Part model, mm, in its own coordinate system. Round coordinates to 2 decimals unless told otherwise and drop trailing zeros. Loops run counter-clockwise (first coordinate to the right, second up) from the corner with the lowest first, then second, coordinate; pieces in that order, holes last. Notation, with made-up numbers: (25, 87) -> (53, 87) arc R19 ccw to (53, 109) -> close; hole circle Ø1 at (-39.75, -38). An arc over 180 degrees is marked (long way). Answer as a JSON object with one key per item and string values. Group by question number.
from build123d import *

# Parameters (mm, degrees)
SKETCH_1_W             = 112
SKETCH_1_H             = 110.77381068
SKETCH_1_R             = 5.25
SM_BASE_FLANGE_1_DEPTH = 6
CHAMFER_1_SIZE         = 15
CUT_EXTRUDE_1_DEPTH    = 10


# Sheet-metal steps are written as plain solids
with BuildPart() as part:
    # Sketch 1 → Базовая кромка1 (new body)
    with BuildSketch(Plane.XY):
        with Locations((0, 58.38690534)):
            Rectangle(SKETCH_1_W, SKETCH_1_H)
        with Locations((-28, 43)):
            Circle(SKETCH_1_R, mode=Mode.SUBTRACT)
        with Locations(Location((28, 73.77381068, 0), (0, 0, 180))):
            Circle(SKETCH_1_R, mode=Mode.SUBTRACT)
        with Locations(Location((28, 43, 0), (0, 0, 180))):
            Circle(SKETCH_1_R, mode=Mode.SUBTRACT)
    extrude(amount=-SM_BASE_FLANGE_1_DEPTH)

    # Фаска1
    chamfer_1_edges = [part.edges().sort_by_distance(p)[0] for p in [
        (56, 3, -3),
        (-56, 3, -3),
        (-56, 113.77381068, -3),
        (56, 113.77381068, -3),
    ]]
    chamfer(chamfer_1_edges, length=CHAMFER_1_SIZE)

    # Sketch 2 → Вырез-Вытянуть1 (cut)
    with BuildSketch(Plane.XY):
        Polygon((-56, 113.77381068), (-56, 86.768448621), (-6.468509112, 113.77381068), align=None)
    extrude(amount=-CUT_EXTRUDE_1_DEPTH, mode=Mode.SUBTRACT)


solid = part.part
Item 1: Two-plate mould, pull along Y, no slides. Class faces 1 (the face through (-31.87, 46.55, -2.96)), 2 (the face through (33.245, 73.543, -2.958)), 3 (the face through (56, 58, -3)), 4 (the face through (-48, 10, -3)): pulls with the +Y half, pulls with the -Y half, needs draft (parallel to the pull), parting line crosses it, or undercut.
Item 2: Band-saw the part on A-A, the plane x = 28. List the corners of the cut face in (y, z).
Item 3: Drill centre lines: line 1 (Y direction, x = 28, z = -4.45); line 2 (Y direction, x = -28, z = -2.9); line 3 (Y direction, x = -45.5, z = -3.95). Where is each one in solid material? Low to high.
Item 4: Band-saw the part on B-B, the plane y = 43. List the corners of the cut face in (x, z), plus the area to 3 significant figures.
Item 5: Band-saw the part on C-C, the plane x = -28. List the corners of the cut face in (y, z).
Item 6: Drop flat-ended pins along their axis: pin 1 Ø3 at (y, z) = (99, -4) entering from +X; pin 2 Ø4 at (x, y) = (-29.5, 41) entering from +Z. Give the stop position or say it passes through.
Item 7: Band-saw the part on D-D, the plane y = 97. List the corners of the cut face in (x, z).
Entries:
{
 "1": {"face 1": "undercut", "face 2": "undercut", "face 3": "needs draft", "face 4": "pulls with the -Y half"},
 "2": {"outline": "(3, -6) -> (37.75, -6) -> (37.75, 0) -> (3, 0) -> close; (48.25, -6) -> (68.52, -6) -> (68.52, 0) -> (48.25, 0) -> close; (79.02, -6) -> (113.77, -6) -> (113.77, 0) -> (79.02, 0) -> close"},
 "3": {"line 1": "3 to 37.75, 48.25 to 68.52, 79.02 to 113.77", "line 2": "3 to 37.75, 48.25 to 102.03", "line 3": "7.5 to 92.49"},
 "4": {"outline": "(-56, -6) -> (-33.25, -6) -> (-33.25, 0) -> (-56, 0) -> close; (-22.75, -6) -> (22.75, -6) -> (22.75, 0) -> (-22.75, 0) -> close; (33.25, -6) -> (56, -6) -> (56, 0) -> (33.25, 0) -> close", "area": "546 mm²"},
 "5": {"outline": "(3, -6) -> (37.75, -6) -> (37.75, 0) -> (3, 0) -> close; (48.25, -6) -> (102.03, -6) -> (102.03, 0) -> (48.25, 0) -> close"},
 "6": {"pin 1": "x = 56", "pin 2": "through"},
 "7": {"outline": "(-37.23, -6) -> (56, -6) -> (56, 0) -> (-37.23, 0) -> close"}
}
